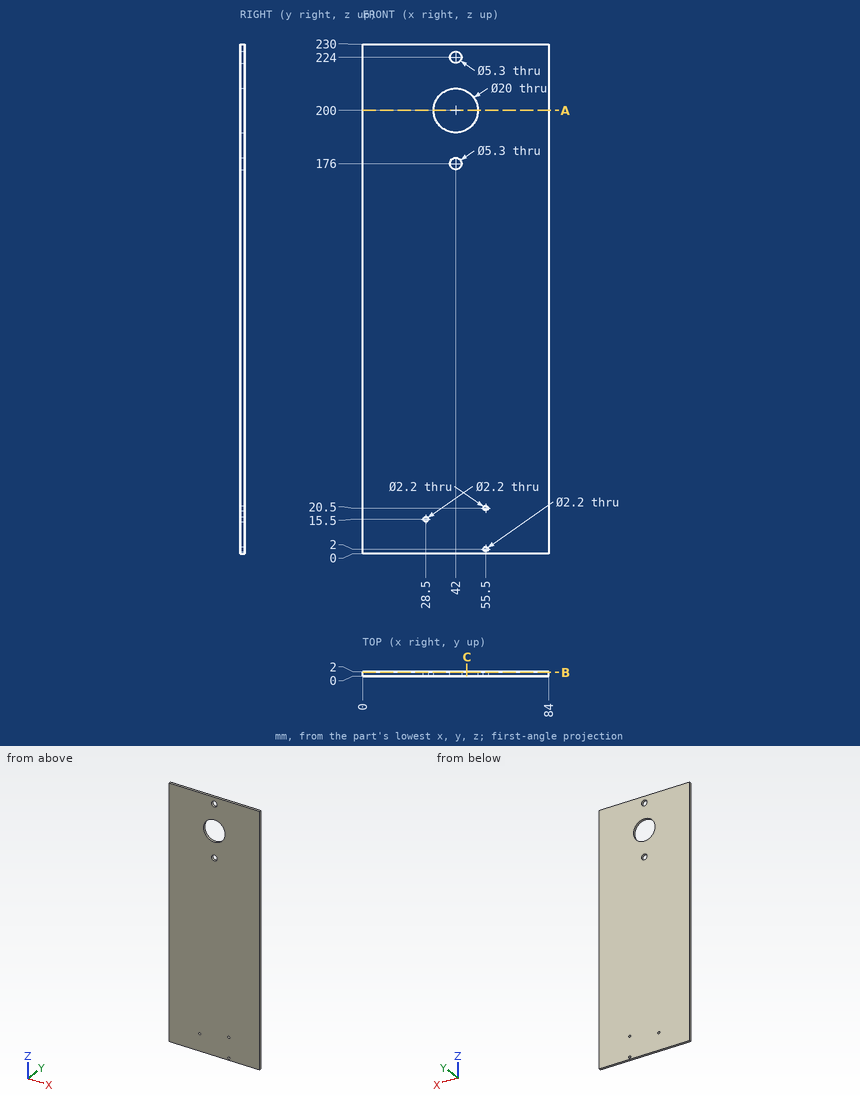
The figure shows three views and two pictorial views of one solid part (mm, origin at its lowest corner). Answer the questions. Give positions to 0.01 mm unless a question says otherwise; leave off trailing zeros. Write each loop counter-clockwise with the first axis right and the second up, starting at its lowest first coordinate (ties: lowest second). Pieces come first, ordered by that corner, then holes.
Q1. The part is cut by section C-C on x = 47. Give the vertices of the cut face in (y, z).
Answer:
outline: (0, 0) - (2, 0) - (2, 191.34) - (0, 191.34) - close; (0, 208.66) - (2, 208.66) - (2, 230) - (0, 230) - close
Q2. Given pin 1 (3.5 mm diameter, centred on x = 28.5, z = 15.5, fed in from -Y), flat-ended and moving along its own axis, determine where the tip first touches the part or whether it passes through.
Answer:
pin 1: stops at y = 0
Q3. Straight lines are drawn through the part: L1, parallel to Z at x = 55.5, y = 1.15; L2, parallel to Z at x = 42, y = 1.15; L3, parallel to X at y = 1.75, z = 175.5. For each, find the intervals that lie inside material, in ascending order.
Answer:
L1: z = 0 to 0.9, 3.1 to 19.4, 21.6 to 230
L2: z = 0 to 173.35, 178.65 to 190, 210 to 221.35, 226.65 to 230
L3: x = 0 to 39.4, 44.6 to 84
Q4. The part is cut by section A-A on z = 200. Give the vertices of the cut face in (x, y), and give its area (3 significant figures).
Answer:
outline: (0, 0) - (32, 0) - (32, 2) - (0, 2) - close; (52, 0) - (84, 0) - (84, 2) - (52, 2) - close
area: 128 mm2
Q5. The part is cut by section B-B on y = 1.65. Give the vertices of the cut face in (x, z), and give its area (3 significant figures).
Answer:
outline: (0, 0) - (84, 0) - (84, 230) - (0, 230) - close; hole circle Ø2.2 at (28.5, 15.5); hole circle Ø20 at (42, 200); hole circle Ø5.3 at (42, 176); hole circle Ø5.3 at (42, 224); hole circle Ø2.2 at (55.5, 2); hole circle Ø2.2 at (55.5, 20.5)
area: 19,000 mm2
